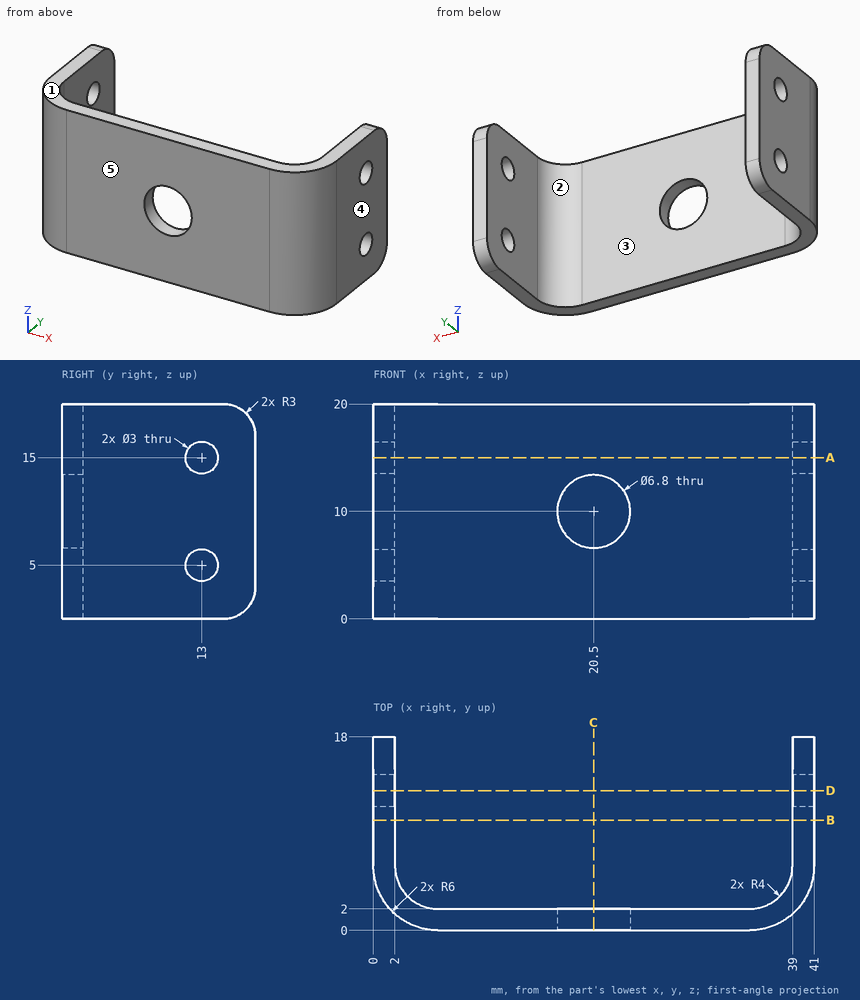
The figure shows three views and two pictorial views of one solid part (mm, origin at its lowest corner). Answer the questions. A direction names the side the tool comes from. Coordinates: 2 decimals unless noted, no trailing zeros. Loops run counter-clockwise (first coordinate to the right, second up) from the corner with the lowest first, then second, coordinate; pieces in that order, holes last. Notation, with made-up numbers: (-21, -36.75) -> (27, -36.75) arc R31 cw to (27, -7.75) -> close; hole circle Ø2 at (67.5, -23.5). An arc over 180 degrees is marked (long way). Write item = value, one per line. Start each with the question number.
1) Given pin 1 Ø8 at (y, z) = (7.5, 10.5) entering from -X; pin 2 Ø3 at (x, z) = (19.5, 14.5) entering from +Y; pin 3 Ø5.5 at (x, z) = (20.5, 10) entering from -Y (3 decimals); pin 4 Ø1.5 at (y, z) = (3, 11.5) entering from +X, each flat-ended and moving along its own axis, determine where each tip first touches the part or whether it passes through.
2) Straight lines are drawn through the part: line 1 (X direction, y = 15.5, z = 11.25); line 2 (Y direction, x = 23.5, z = 17.5); line 3 (Y direction, x = 0.95, z = 15). For each, find the intervals that lie inside material, in ascending order. Write a range as from..to.
3) A cutting plane is placed at C-C (x = 20.5). Give the vertices of the cut face in (y, z), then the cut area to 3 significant figures.
4) A cutting plane is placed at D-D (y = 13). Give the vertices of the cut face in (x, z), then the cut area to 3 significant figures.
5) A tool of negligible diameter and unlimited length cuts with its end or side. For the marked faces 1 and 2, from which of +Z, -Z, +X, -X, +Y, -Y can it reach the whole face along a straight path? Write none if from no direction.
6) The mould has two halves that part along X. Classify the marked faces 3, 4 and 5: released by +X, released by -X, zero draft, split by the parting line, or undercut.
7) A cutting plane is placed at B-B (y = 10.25). Give the vertices of the cut face in (x, z).
8) A cutting plane is placed at A-A (z = 15). Give the vertices of the cut face in (x, y).
Responses:
q1.pin_1 = 0
q1.pin_2 = 2
q1.pin_3 = through
q1.pin_4 = 40.56
q2.line_1 = 0..2, 39..41
q2.line_2 = 0..2
q2.line_3 = 2.76..11.5, 14.5..18
q3.outline = (0, 0) -> (2, 0) -> (2, 6.6) -> (0, 6.6) -> close; (0, 13.4) -> (2, 13.4) -> (2, 20) -> (0, 20) -> close
q3.area = 26.4 mm²
q4.outline = (0, 0) -> (2, 0) -> (2, 3.5) -> (0, 3.5) -> close; (0, 6.5) -> (2, 6.5) -> (2, 13.5) -> (0, 13.5) -> close; (0, 16.5) -> (2, 16.5) -> (2, 20) -> (0, 20) -> close; (39, 0) -> (41, 0) -> (41, 3.5) -> (39, 3.5) -> close; (39, 6.5) -> (41, 6.5) -> (41, 13.5) -> (39, 13.5) -> close; (39, 16.5) -> (41, 16.5) -> (41, 20) -> (39, 20) -> close
q4.area = 56.0 mm²
q5.face_1 = +Z, +X, -X, +Y, -Y
q5.face_2 = +Z, -Z, +Y
q6.face_3 = undercut
q6.face_4 = released by +X
q6.face_5 = zero draft
q7.outline = (0, 0) -> (2, 0) -> (2, 20) -> (0, 20) -> close; (39, 0) -> (41, 0) -> (41, 20) -> (39, 20) -> close
q8.outline = (0, 6) arc R6 ccw to (6, 0) -> (35, 0) arc R6 ccw to (41, 6) -> (41, 11.5) -> (39, 11.5) -> (39, 6) arc R4 cw to (35, 2) -> (6, 2) arc R4 cw to (2, 6) -> (2, 11.5) -> (0, 11.5) -> close; (0, 14.5) -> (2, 14.5) -> (2, 18) -> (0, 18) -> close; (39, 14.5) -> (41, 14.5) -> (41, 18) -> (39, 18) -> close
